```python
from build123d import *

# Parameters (mm, degrees)
SKETCH1_R           = 73.025
SKETCH1_R_2         = 70.485
BOSS_EXTRUDE1_DEPTH = 1.016
SKETCH1_3_R         = 2.54
SKETCH1_3_R_2       = 1.651
BOSS_EXTRUDE2_DEPTH = 1.016
SKETCH1_4_R         = 1.651
CUT_EXTRUDE1_DEPTH  = 1.016
CIRPATTERN2_COUNT   = 12


with BuildPart() as part:
    # Sketch1 → Boss-Extrude1 (new body)
    with BuildSketch(Plane(origin=(0, 0, 0), x_dir=(1, 0, 0), z_dir=(0, 1, 0))):
        with Locations(Location((0, 0, 0), (0, 0, 270))):
            Circle(SKETCH1_R)
        with Locations(Location((0, 0, 0), (0, 0, 270))):
            Circle(SKETCH1_R_2, mode=Mode.SUBTRACT)
    extrude(amount=BOSS_EXTRUDE1_DEPTH)

    # Sketch1<3> → Boss-Extrude2 (add)
    with BuildSketch(Plane(origin=(0, 0, 0), x_dir=(1, 0, 0), z_dir=(0, 1, 0))):
        with Locations((0, -71.755)):
            Circle(SKETCH1_3_R)
        with Locations((0, -71.755)):
            Circle(SKETCH1_3_R_2, mode=Mode.SUBTRACT)
    boss_extrude2 = extrude(amount=BOSS_EXTRUDE2_DEPTH)

    # Sketch1<4> → Cut-Extrude1 (cut)
    with BuildSketch(Plane(origin=(0, 0, 0), x_dir=(1, 0, 0), z_dir=(0, 1, 0))):
        with Locations(Location((0, -71.755, 0), (0, 0, 270))):
            Circle(SKETCH1_4_R)
    cut_extrude1 = extrude(amount=CUT_EXTRUDE1_DEPTH, mode=Mode.SUBTRACT)

    # CirPattern2: Boss-Extrude2, Cut-Extrude1 ×12 about axis
    cirpattern2_axis = Axis((0, 0, 0), (0, 1, 0))
    add([boss_extrude2.rotate(cirpattern2_axis, i * 360 / CIRPATTERN2_COUNT) for i in range(1, CIRPATTERN2_COUNT)])
    add([cut_extrude1.rotate(cirpattern2_axis, i * 360 / CIRPATTERN2_COUNT) for i in range(1, CIRPATTERN2_COUNT)], mode=Mode.SUBTRACT)


solid = part.part
```
Model file for the job. Use its own axes, mm. A direction names the side the tool comes from. Round coordinates to 2 decimals unless told otherwise and drop trailing zeros. Write each loop counter-clockwise with the first axis right and the second up, starting at its lowest first coordinate (ties: lowest second). Pieces come first, ordered by that corner, then holes. Notation, with made-up numbers: (6.5, 1.25) - (27.5, 1.25) arc R9 ccw to (27.5, 15.25) - close; hole circle Ø4 at (2, 68). An arc over 180 degrees is marked (long way). Use CSV: the item, a comma, the result in double quotes. Start each with the question number.
Item 1: Band-saw the part on A-A (x = -15.5). Write the cut outline in (y, z), and give its area (3 significant figures).
Item 2: Tool access for faces 4 (the face through (51.47, 0.5, 51.8)), 5 (the face through (-49.68, 0.5, -50)): list every direction of +Z, -Z, +X, -X, +Y, -Y with a clear straight run to the whole face (end or side of a thin tool).
Item 3: Band-saw the part on B-B (z = 24). Write the cut outline in (x, y).
Item 4: Drill centre lines: L1, parallel to X at y = 0.3, z = -36; L2, parallel to X at y = 0.7, z = 0 (3 decimals); L3, parallel to X at y = 0.15, z = -10. Where is each one in solid material? Low to high. Write a range as [from, to].
Item 5: Two-plate mould, pull along X, no slides. Class faces 1 (the face through (70.475, 0.501, 19.129)), 2 (the face through (36.232, 0.501, -63.754)), 3 (the face through (-51.47, 0.5, -51.8)): released by +X, released by -X, zero draft, split by the parting line, or undercut.
Item 6: Band-saw the part on C-C (y = 0.7). State how many separate pieces and enclosed holes the cut face has, and give its area (3 significant figures).
Checked values:
1,outline,"(0, -71.36) - (1.02, -71.36) - (1.02, -68.76) - (0, -68.76) - close; (0, 68.76) - (1.02, 68.76) - (1.02, 71.36) - (0, 71.36) - close"
1,area,"5.29 mm²"
2,face 4,"+Z, +X, +Y, -Y"
2,face 5,"+Y, -Y"
3,outline,"(-68.97, 0) - (-66.27, 0) - (-66.27, 1.02) - (-68.97, 1.02) - close; (66.27, 0) - (68.97, 0) - (68.97, 1.02) - (66.27, 1.02) - close"
4,L1,"x = [-64.68, -63.79], [-60.5, -59.6], [59.6, 60.5], [63.79, 64.68]"
4,L2,"x = [-74.295, -73.406], [-70.104, -69.215], [69.215, 70.104], [73.406, 74.295]"
4,L3,"x = [-72.34, -69.77], [69.77, 72.34]"
5,face 1,"released by +X"
5,face 2,"undercut"
5,face 3,"released by -X"
6,separate pieces,"1"
6,enclosed holes,"13"
6,area,"1,140 mm²"
